```python
from build123d import *

# Parameters (mm, degrees)
SKETCH_2_W          = 104
SKETCH_2_H          = 163
EXTRUDE_1_DEPTH     = 4
SKETCH_4_W          = 104
SKETCH_4_H          = 29.5
SKETCH_4_H_2        = 20.5
CUT_EXTRUDE_1_DEPTH = 4
SKETCH_5_W          = 4
SKETCH_5_H          = 50
EXTRUDE_2_DEPTH     = 4
SKETCH_7_W          = 4
SKETCH_7_H          = 50
EXTRUDE_3_DEPTH     = 4


with BuildPart() as part:
    # 스케치2 → 보스-돌출1 (new body)
    with BuildSketch(Plane.XY.offset(40)):
        with Locations((-56, 1.5)):
            Rectangle(SKETCH_2_W, SKETCH_2_H)
    extrude(amount=EXTRUDE_1_DEPTH)

    # 스케치4 → 컷-돌출1 (cut)
    with BuildSketch(Plane(origin=(0, 0, 40), x_dir=(-1, 0, 0), z_dir=(0, 0, -1))):
        with Locations((56, 68.25)):
            Rectangle(SKETCH_4_W, SKETCH_4_H)
        with Locations((56, -69.75)):
            Rectangle(SKETCH_4_W, SKETCH_4_H_2)
    extrude(amount=-CUT_EXTRUDE_1_DEPTH, mode=Mode.SUBTRACT)

    # 스케치5 → 보스-돌출2 (add)
    with BuildSketch(Plane.ZY.offset(108)):
        with Locations((42, -3)):
            Rectangle(SKETCH_5_W, SKETCH_5_H)
    extrude(amount=EXTRUDE_2_DEPTH)

    # 스케치7 → 보스-돌출3 (add)
    with BuildSketch(Plane(origin=(-4, 0, 0), x_dir=(0, 0, -1), z_dir=(1, 0, 0))):
        with Locations((-42, -3)):
            Rectangle(SKETCH_7_W, SKETCH_7_H)
    extrude(amount=EXTRUDE_3_DEPTH)


solid = part.part
```
For this review, take the finished solid that the model builds, in its own axes (mm). A direction names the side the tool comes from. Round coordinates to 2 decimals unless told otherwise and drop trailing zeros. Write each loop counter-clockwise with the first axis right and the second up, starting at its lowest first coordinate (ties: lowest second). Pieces come first, ordered by that corner, then holes. Notation, with made-up numbers: (30, 59) -> (62, 59) arc R10 ccw to (62, 75) -> close; hole circle Ø2 at (63, 59). An arc over 180 degrees is marked (long way). Use one line per item in the form item = value.
1) Tool access review of faces 1 (the flat face through (-4, 38, 42)), 2 (the flat face through (-108, 38, 42)), 3 (the flat face through (-108, -44, 42)): name each direction out of +Z, -Z, +X, -X, +Y, -Y from which nothing blocks a thin tool from reaching the whole face with its end or side.
Found:
face_1 = +Z, -Z, +X, +Y
face_2 = +Z, -Z, -X, +Y
face_3 = +Z, -Z, -X, -Y
2) Clearance check with flat-ended pins moving along their axes: pin 1 (2 mm diameter, centred on x = -110, z = 41.5, fed in from -Y); pin 2 (2 mm diameter, centred on y = -45, z = 42, fed in from +X); pin 3 (1.2 mm diameter, centred on y = -48, z = 42, fed in from -X). State where each tip first meets the part, or that it passes through.
Found:
pin_1 = -28
pin_2 = -4
pin_3 = -108
3) Take a section at B-B, the plane y = -33. Write out the cut boundary in (x, z), and give its area (3 significant figures).
Found:
outline = (-108, 40) -> (-4, 40) -> (-4, 44) -> (-108, 44) -> close
area = 416 mm2
4) To check wall thickness, follow L1, parallel to X at y = -31, z = 42.85. State the ranges of the line that lie inside material, in increasing order. Write a range as from..to.
Found:
L1 = -108..-4
5) Take a section at A-A, the plane z = 40.7. Write out the cut boundary in (x, y), and give its area (3 significant figures).
Found:
outline = (-112, -28) -> (-108, -28) -> (-108, -59.5) -> (-4, -59.5) -> (-4, -28) -> (0, -28) -> (0, 22) -> (-4, 22) -> (-4, 53.5) -> (-108, 53.5) -> (-108, 22) -> (-112, 22) -> close
area = 12,200 mm2
